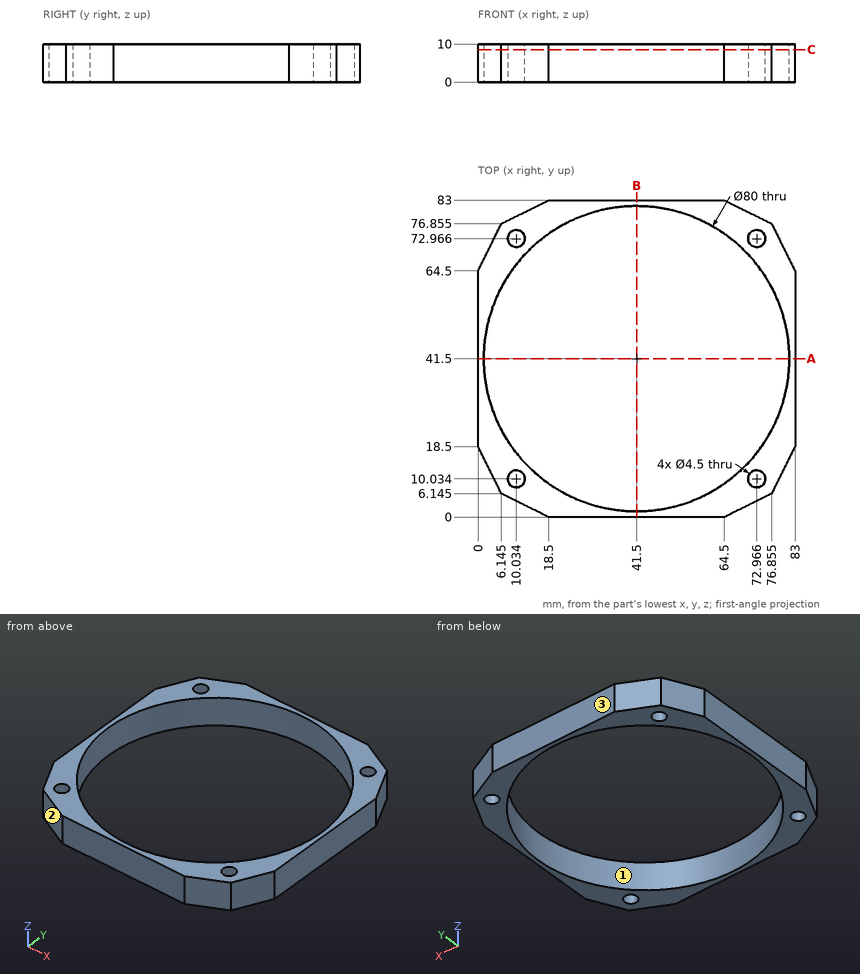
The figure shows three views and two pictorial views of one solid part (mm, origin at its lowest corner). Answer the questions. Coordinates: 2 decimals unless noted, no trailing zeros. Loops run counter-clockwise (first coordinate to the right, second up) from the corner with the lowest first, then second, coordinate; pieces in that order, holes last. Notation, with made-up numbers: (-39.5, -34) - (-21.5, -34) arc R23 cw to (-21.5, -10) - close; hole circle Ø7 at (-24.5, -33.5). An arc over 180 degrees is marked (long way). Write item = value, one per line.
1) Section A-A (y = 41.5) is taken. Determine the outline of the cut face in (x, z).
Responses:
outline = (0, 0) - (1.5, 0) - (1.5, 10) - (0, 10) - close; (81.5, 0) - (83, 0) - (83, 10) - (81.5, 10) - close
2) Each of these flat-tipped pins is pushed along its axis until it touches: P1, Ø7, axis at x = 72.97, y = 10.03, coming from the -Z side; P2, Ø2, axis at y = 67.5, z = 8.5, coming from the -X side (1 decimal). Where does it stop, or does it pass through?
Responses:
P1 = 0
P2 = 1
3) Determine the mould class of the marked faces 1, 2 and 3 for opening direction Y: pulls with the +Y half, pulls with the -Y half, needs draft (parallel to the pull), parting line crosses it, or undercut.
Responses:
face_1 = undercut
face_2 = pulls with the -Y half
face_3 = pulls with the +Y half
4) Find the intervals of material crossed by line 1 along Y through (x, z) = (74.5, 4) (1 decimal); line 2 along X through (y, z) = (75, 7.75) (1 decimal); line 3 along X through (y, z) = (41.5, 3.25), in increasing order.
Responses:
line_1 = 5 to 8.4, 11.7 to 18.9, 64.1 to 71.3, 74.6 to 78
line_2 = 5.2 to 9.1, 11 to 19.6, 63.4 to 72, 73.9 to 77.8
line_3 = 0 to 1.5, 81.5 to 83
5) Section C-C (z = 8.5) is taken. Count the separate pieces of the cut face and the enclosed holes in it, plus the area to 3 significant figures.
Responses:
separate_pieces = 1
enclosed_holes = 5
area = 1,340 mm^2
